Can you work these out from the model? Positions are in its coordinate system, mm. Face numbers are marked on the shaded views. A direction names the side the tool comes from. Give positions to 0.01 mm unless a question says otherwise; leave off trailing zeros. Order: outer loops, then holes, each group sorted by start corner. A loop starts at its lowest first (then second) coordinate and runs counter-clockwise, first axis right, second up. Notation, with made-up numbers: (35, -15.75) - (50, -15.75) arc R19 ccw to (50, 19.25) - close; hole circle Ø1 at (10, 21). An arc over 180 degrees is marked (long way). One line per question, with ' | ' between items.
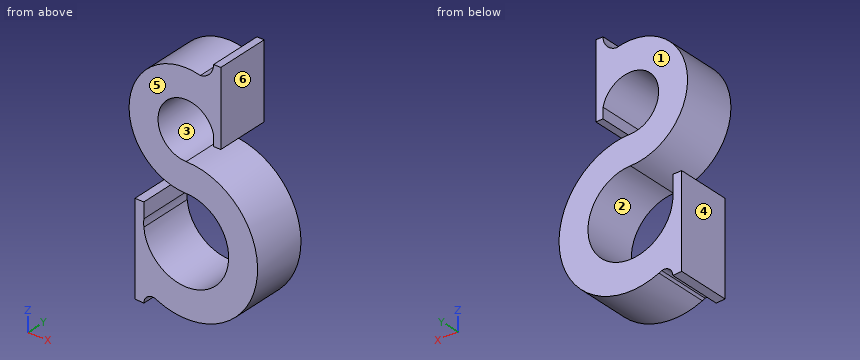
```python
from build123d import *

# Parameters (mm, degrees)
F1_DEPTH = 38.1


with BuildPart() as f1:
    # F0 (on Front) → F1 (new body)
    with BuildSketch(Plane.XZ):
        with BuildLine():
            ThreePointArc((-20.02527, -96.13909), (49.101263, -60.382661), (0, 0))
            ThreePointArc((0, 0), (-15.465639, 32.071315), (19.259737, 24.20344))
            Line((19.259737, 24.20344), (19.259737, 54.919144))
            ThreePointArc((19.259737, 54.919144), (14.720483, 57.04847), (9.950919, 58.594471))
            ThreePointArc((9.950919, 58.594471), (-39.769695, 24.779488), (0, -20.32))
            ThreePointArc((0, -20.32), (22.020464, -70.285545), (-29.715391, -52.825367))
            Line((-29.715391, -52.825367), (-29.715391, -90.559729))
            ThreePointArc((-29.715391, -90.559729), (-25.941689, -93.080237), (-21.955613, -95.249332))
            ThreePointArc((-21.955613, -95.249332), (-20.951886, -95.610565), (-20.02527, -96.13909))
        make_face()
        Polygon((19.259737, 54.919144), (19.259737, 24.20344), (19.259737, 16.724238), (24.339737, 16.724238), (24.339737, 69.048567), (19.259737, 69.048567), align=None)
        with BuildLine():
            Line((-29.715391, -101.220826), (-29.715391, -90.559729))
            Line((-29.715391, -90.559729), (-29.715391, -52.825367))
            ThreePointArc((-29.715391, -52.825367), (-29.835124, -50.155124), (-29.715391, -47.484882))
            Line((-29.715391, -47.484882), (-29.715391, -36.713058))
            Line((-29.715391, -36.713058), (-35.986979, -36.713058))
            Line((-35.986979, -36.713058), (-35.986979, -100.922184))
            Line((-35.986979, -100.922184), (-29.715391, -101.220826))
        make_face()
        with BuildLine():
            ThreePointArc((-29.715391, -101.220826), (-27.305323, -96.325091), (-21.955613, -95.249332))
            ThreePointArc((-21.955613, -95.249332), (-25.941689, -93.080237), (-29.715391, -90.559729))
            Line((-29.715391, -90.559729), (-29.715391, -101.220826))
        make_face()
        with BuildLine():
            ThreePointArc((9.950919, 58.594471), (14.720483, 57.04847), (19.259737, 54.919144))
            Line((19.259737, 54.919144), (19.259737, 69.048567))
            ThreePointArc((19.259737, 69.048567), (16.59525, 62.049598), (9.950919, 58.594471))
        make_face()
    extrude(amount=F1_DEPTH)


solid = f1.part
```
(1) If I drill on line 1 (Z direction, x = 12, y = -4.5); line 2 (Z direction, x = 14.5, y = -17.5); line 3 (X direction, y = -22, z = -73.5), over which ranges is the centre line in solid material (lowest first)?
Answer below:
line 1: -98.85 to -77.47, -22.84 to -1.46, 35.47 to 59.04 | line 2: -98.17 to -76.23, -24.08 to -2.14, 33.2 to 60.24 | line 3: -35.99 to -18.58, 18.58 to 44.39
(2) Will these pins go through, and if not, where does the flat tip stop? pin 1 (2 mm diameter, centred on x = 20, z = -3, fed in from -Y); pin 2 (5.5 mm diameter, centred on y = -13, z = -40, fed in from +X); pin 3 (1.5 mm diameter, centred on x = 22, y = -27, fed in from -Z); pin 4 (3 mm diameter, centred on y = -12.5, z = -8, fed in from +X).
Answer below:
pin 1: through | pin 2: x = 49.61 | pin 3: z = -95.59 | pin 4: x = 29.37
(3) Imagine slicing it at B-B (z = -73). List the corners of the cut face in (x, y) for me.
Answer below:
outline: (-35.99, -38.1) - (-19.19, -38.1) - (-19.19, 0) - (-35.99, 0) - close; (19.19, -38.1) - (44.65, -38.1) - (44.65, 0) - (19.19, 0) - close
(4) Imagine slicing it at C-C (y = -35.5). List the corners of the cut face in (x, z) for me.
Answer below:
outline: (-35.99, -100.92) - (-29.72, -101.22) arc R6.18 cw to (-21.96, -95.25) arc R6.18 cw to (-20.03, -96.14) arc R50.16 ccw (long way) to (0, 0) arc R19.76 cw (long way) to (19.26, 24.2) - (19.26, 16.72) - (24.34, 16.72) - (24.34, 69.05) - (19.26, 69.05) arc R10.52 cw to (9.95, 58.59) arc R40.08 ccw (long way) to (0, -20.32) arc R29.84 cw (long way) to (-29.72, -52.83) arc R29.84 cw to (-29.72, -47.48) - (-29.72, -36.71) - (-35.99, -36.71) - close
(5) Imagine slicing it at D-D (x = -24). List the corners of the cut face in (y, z) for me.
Answer below:
outline: (-38.1, -95.06) - (0, -95.06) - (0, -67.88) - (-38.1, -67.88) - close; (-38.1, -12.34) - (0, -12.34) - (0, 51.87) - (-38.1, 51.87) - close
(6) On a 3-axis mill with a long thin cutter (end or side, diameter ignored), from which of +Z, -Z, +X, -X, +Y, -Y can I reach the whole of each face in a straight line? I mean the marked faces 5 and 6. Say none if no direction works.
Answer below:
face 5: +Z, -Z, +X, -X, -Y | face 6: +Z, +X, +Y, -Y
(7) If we mould it in two halves opening along X, with no side actions, what happens to the marked faces 1, 2, 3 and 4? For each: released by +X, released by -X, zero draft, split by the parting line, or undercut.
Answer below:
face 1: zero draft | face 2: undercut | face 3: undercut | face 4: released by -X
(8) Imagine slicing it at A-A (x = 0). List the corners of the cut face in (y, z) for me.
Answer below:
outline: (-38.1, -100.31) - (0, -100.31) - (0, -79.99) - (-38.1, -79.99) - close; (-38.1, -20.32) - (0, -20.32) - (0, 0) - (-38.1, 0) - close; (-38.1, 39.53) - (0, 39.53) - (0, 59.85) - (-38.1, 59.85) - close
